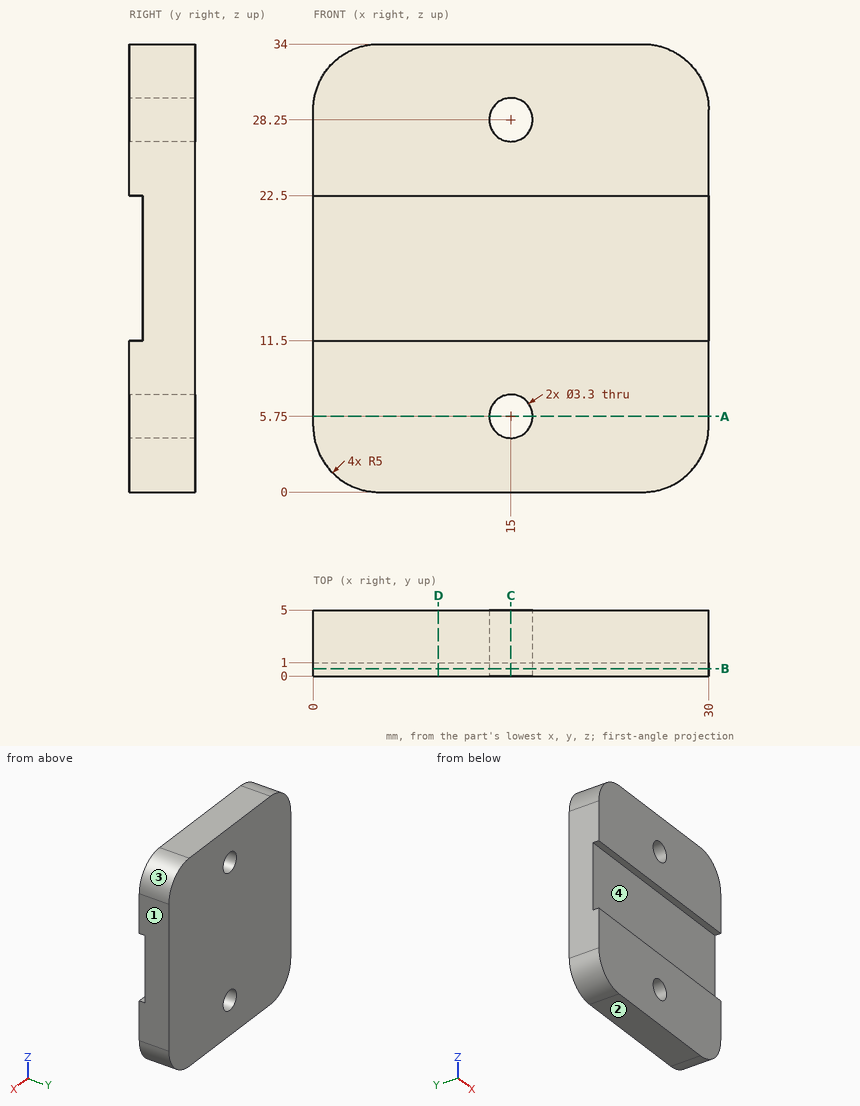
Could you check a few things on this drawing? It's one solid part, dimensions in mm from its lowest x, y, z. Round coordinates to 2 decimals unless told otherwise and drop trailing zeros. Write each loop counter-clockwise with the first axis right and the second up, starting at its lowest first coordinate (ties: lowest second). Pieces come first, ordered by that corner, then holes.
Q1. If we section it at A-A on z = 5.75: Write out the boundary of the cut face in (x, y).
Q2. If we section it at B-B on y = 0.55: Write out the boundary of the cut face in (x, z), plus the area to 3 significant figures.
Q3. If we section it at D-D on x = 9.5: Write out the boundary of the cut face in (y, z), plus the area to 3 significant figures.
Q4. If we section it at C-C on x = 15: Write out the boundary of the cut face in (y, z).
Q5. If we mould it in two halves opening along Z, with no side actions, what happens to the marked faces 1, 2, 3 and 4? For each: +Z half, -Z half, draft (parallel to the pull), parting line (faces both ways), or undercut.
Q6. Please list where these lines run through material, in increasing order: probe 1 along Z at (x, y) = (15, 1.15); probe 2 along Z at (x, y) = (10, 0.45); probe 3 along Y at (x, z) = (13.5, 18.5).
Q7. Will this pin go through, and if not, where does the flat tip stop? P1, Ø1, axis at x = 18, z = 13, coming from the -Y side.
Answer below:
1. outline: (0, 0) - (13.35, 0) - (13.35, 5) - (0, 5) - close; (16.65, 0) - (30, 0) - (30, 5) - (16.65, 5) - close
2. outline: (0, 5) arc R5 ccw to (5, 0) - (25, 0) arc R5 ccw to (30, 5) - (30, 11.5) - (0, 11.5) - close; (0, 22.5) - (30, 22.5) - (30, 29) arc R5 ccw to (25, 34) - (5, 34) arc R5 ccw to (0, 29) - close; hole circle Ø3.3 at (15, 5.75); hole circle Ø3.3 at (15, 28.25)
2. area: 651 mm2
3. outline: (0, 0) - (5, 0) - (5, 34) - (0, 34) - (0, 22.5) - (1, 22.5) - (1, 11.5) - (0, 11.5) - close
3. area: 159 mm2
4. outline: (0, 0) - (5, 0) - (5, 4.1) - (0, 4.1) - close; (0, 7.4) - (5, 7.4) - (5, 26.6) - (0, 26.6) - (0, 22.5) - (1, 22.5) - (1, 11.5) - (0, 11.5) - close; (0, 29.9) - (5, 29.9) - (5, 34) - (0, 34) - close
5. face 1: draft
5. face 2: -Z half
5. face 3: +Z half
5. face 4: undercut
6. probe 1: z = 0 to 4.1, 7.4 to 26.6, 29.9 to 34
6. probe 2: z = 0 to 11.5, 22.5 to 34
6. probe 3: y = 1 to 5
7. P1: stops at y = 1
